Input: part model. Units: mm. Frame: model coordinates. A direction names the side the tool comes from. Coordinates: 2 decimals unless noted, no trailing zeros. Order: outer loops, then holes, each group sorted by start corner. A loop starts at its lowest first (then second) coordinate and runs counter-clockwise, first axis right, second up. Notation, with made-up numbers: (53.25, -3.75) -> (86.25, -3.75) arc R23 ccw to (86.25, 14.25) -> close; hole circle Ø6 at (57, 13.5). An arc over 180 degrees is marked (long way). Use one line per item in the form item = value. Start each with the question number.
1) Section query A-A on x = 0. Output: boundary loops of the cut face in (y, z), then the cut area to 3 significant figures.
2) Draft query along X for faces 4 (the cylindrical face through (1.32, 30.97, 3.75)), 5 (the flat face through (11, -5, -1.5)), 6 (the flat face through (0, -25, 3)), 7 (the cylindrical face through (-14.47, -1.43, 1.23)). Return one class per face: pulls with the +X half, pulls with the -X half, needs draft (parallel to the pull), parting line crosses it, or undercut.
3) Access query for faces 1 (the flat face through (-19, 0, 0)), 2 (the flat face through (-3, -28, 3)), 3 (the flat face through (0, -13, 4)). Directions: +Z, -Z, +X, -X, +Y, -Y. A direction counts if a zero-diameter tool reaches every point of the face in a straight line with its end or side. Return the directions, or none.
4) Ray query, line 1 along Y through (x, z) = (-19, 1.95); line 2 along Y through (x, z) = (-19, 1.85); line 3 along Z through (x, y) = (-18, -6). Return the intervals inside material, ascending.
5) Section query B-B on z = 0.85. Output: boundary loops of the cut face in (x, y), then the cut area to 3 significant figures.
6) Pin query (flat end, axial travel): pin 1 (10.5 mm diameter, centred on x = 18, y = 0.5, fed in from +Z); pin 2 (4.5 mm diameter, centred on x = 19, y = -1, fed in from +Z); pin 3 (1.2 mm diameter, centred on x = -1.5, z = 3.5, fed in from -Y); pin 4 (18.5 mm diameter, centred on x = 0, y = 0, fed in from +Z). Return the tip coordinate at first contact, or that it passes through.
from build123d import *
from build123d import SkipClean  # not in build123d's __all__

# Parameters (mm, degrees)
F0_R     = 31
F0_R_2   = 11.5
F1_DEPTH = 1.5
F2_R     = 31
F2_R_2   = 4.75
F2_R_3   = 11.5
F3_DEPTH = 4
F5_DEPTH = 1.5


# Not quite as in the source:
# - a fillet or chamfer that OpenCascade refuses, or shapes differently, is made with other operations: its cross-section is extruded or revolved along the edge and cut away or added


with BuildPart() as f1:
    # F0 (on Top) → F1 (new body)
    with BuildSketch(Plane.XY):
        Circle(F0_R)
        Circle(F0_R_2, mode=Mode.SUBTRACT)
    extrude(amount=-F1_DEPTH)

    # F2 (on face) → F3 (join)
    with BuildSketch(Plane(origin=(0, 0, -1.5), x_dir=(1, 0, 0), z_dir=(0, 0, -1))):
        Circle(F2_R)
        with Locations((-19, 0)):
            Circle(F2_R_2, mode=Mode.SUBTRACT)
        Circle(F2_R_3, mode=Mode.SUBTRACT)
        with Locations((19, 0)):
            Circle(F2_R_2, mode=Mode.SUBTRACT)
    extrude(amount=-F3_DEPTH)

    # F4 (on face) → F5 (join)
    with BuildSketch(Plane.XY.offset(2.5)):
        with BuildLine():
            ThreePointArc((3, -30.8544972411), (22.9564805665, -20.832666656), (31, 0))
            ThreePointArc((31, 0), (-20.832666656, 22.9564805665), (-3, -30.8544972411))
            Line((-3, -30.8544972411), (-3, -25))
            Line((-3, -25), (3, -25))
            Line((3, -25), (3, -30.8544972411))
        make_face()
        with BuildLine():
            ThreePointArc((-11.4901151316, 0.4767119288), (0, 11.5), (11.4901151316, 0.4767119288))
            ThreePointArc((11.4901151316, 0.4767119288), (19.2384757484, 7.5212202678), (26.525, 0))
            ThreePointArc((26.525, 0), (19.2384757484, -7.5212202678), (11.4901151316, -0.4767119288))
            ThreePointArc((11.4901151316, -0.4767119288), (0, -11.5), (-11.4901151316, -0.4767119288))
            ThreePointArc((-11.4901151316, -0.4767119288), (-26.525, 0), (-11.4901151316, 0.4767119288))
        make_face(mode=Mode.SUBTRACT)
    with SkipClean():  # cleaning this boolean's faces spoils the solid; the shape is the same uncleaned
        extrude(amount=F5_DEPTH)

    # F6: fillet of radius 5 on 1 edges, made by hand

    # F6_s1 → F6_t2 (revolve, cut)
    with BuildSketch(Plane.XZ):
        with BuildLine():
            ThreePointArc((31, 3.5), (29.5355339059, -0.0355339059), (26, -1.5))
            Line((26, -1.5), (31, -1.5))
            Line((31, -1.5), (31, 3.5))
        make_face()
    revolve(axis=Axis((0, 0, -1.5), (0, 0, 1)), mode=Mode.SUBTRACT)


solid = f1.part
Answers below:
q1.outline = (-30.9, 2.5) arc R5 ccw to (-26, -1.5) -> (-11.5, -1.5) -> (-11.5, 4) -> (-25, 4) -> (-25, 2.5) -> close; (11.5, -1.5) -> (26, -1.5) arc R5 ccw to (31, 3.5) -> (31, 4) -> (11.5, 4) -> close
q1.area = 195 mm^2
q2.face_4 = parting line crosses it
q2.face_5 = needs draft
q2.face_6 = undercut
q2.face_7 = undercut
q3.face_1 = +Z
q3.face_2 = +Z, -Y
q3.face_3 = +Z, +X, -X, +Y, -Y
q4.line_1 = -24.18 to -4.75, 4.75 to 24.18
q4.line_2 = -24.14 to -4.75, 4.75 to 24.14
q4.line_3 = -1.5 to 2.5
q5.outline = circle Ø60.48 at (0, 0); hole circle Ø9.5 at (-19, 0); hole circle Ø23 at (0, 0); hole circle Ø9.5 at (19, 0)
q5.area = 2,320 mm^2
q6.pin_1 = 2.5
q6.pin_2 = 0
q6.pin_3 = -25
q6.pin_4 = through
